```python
from build123d import *

# Parameters (mm, degrees)
F0_W           = 50.8
F0_H           = 43.18
F1_DEPTH       = 50.8
F3_D           = 6.35
F3_CBORE_D     = 9.525
F3_CBORE_DEPTH = 6.35
F5_D           = 7.9375
F6_SIZE        = 3.175


with BuildPart() as f1:
    # F0 (on Front) → F1 (new body)
    with BuildSketch(Plane.XZ):
        with Locations((25.4, -21.59)):
            Rectangle(F0_W, F0_H)
    extrude(amount=-F1_DEPTH)

    # F3 (through all)
    with Locations(Plane.XY):
        with Locations((7.1374, 7.1628), (7.1374, 43.6626), (43.6372, 43.6626), (43.6372, 7.1628)):
            CounterBoreHole(F3_D / 2, F3_CBORE_D / 2, F3_CBORE_DEPTH)

    # F5 (through all)
    with Locations(Plane.XY):
        with Locations((26.850944, 26.850944), (26.850944, 45.138944)):
            Hole(F5_D / 2)

    # F6
    f6_edges = [f1.edges().sort_by_distance(p)[0] for p in [
        (50.8, 50.8, -21.59),
        (50.8, 0, -21.59),
        (0, 50.8, -21.59),
        (0, 0, -21.59),
    ]]
    chamfer(f6_edges, length=F6_SIZE)


solid = f1.part
```
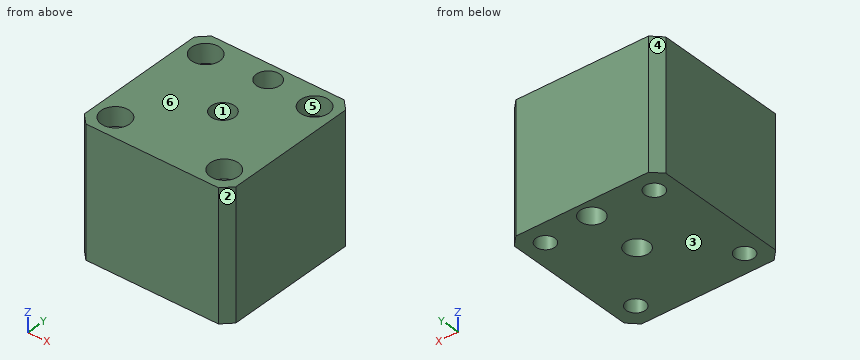
Read the model definition and answer for the solid it produces. Units are mm, in the model's axes. Face numbers are marked on the shaded views. A direction names the side the tool comes from. Coordinates: 2 decimals unless noted, no trailing zeros. Write each loop counter-clockwise with the first axis right and the second up, starting at its lowest first coordinate (ties: lowest second). Pieces come first, ordered by that corner, then holes. Notation, with made-up numbers: (-23.5, 81) - (-18.5, 81) arc R21 cw to (-18.5, 88) - close; hole circle Ø6 at (57.25, 31). An arc over 180 degrees is marked (long way). Answer as a JSON object with one key per item and string values. Group by question number.
1. A cutting plane is placed at B-B (z = -21). Give the number of separate pieces and of enclosed holes in the cut face, plus the area to 3 significant figures.
2. Which of the six approach directions +Z, -Z, +X, -X, +Y, -Y give full straight-line access (tool end or side, diameter ignored) to the marked faces 5 and 6?
3. A cutting plane is placed at A-A (x = 29.5). Determine the outline of the cut face in (y, z), plus the area to 3 significant figures.
4. Consider L1, parallel to X at y = 7, z = -36; L2, parallel to Y at x = 44.5, z = -13; L3, parallel to Y at x = 28.5, z = -27. Determine where each line is inside the solid, lowest interval first. Write a range as [from, to].
5. A cutting plane is placed at D-D (x = 9.5). Determine the outline of the cut face in (y, z), plus the area to 3 significant figures.
6. Each of these flat-tipped pins is pushed along its axis until it touches: P1, Ø9, axis at x = 26.85, y = 45.14, coming from the +Z side; P2, Ø3, axis at x = 6, y = 9, coming from the +Z side. Where does it stop, or does it pass through?
7. The mould has two halves that part along Y. Classify the marked faces 1, 2, 3 and 4: +Y half, -Y half, draft (parallel to the pull), parting line (faces both ways), or undercut.
8. A cutting plane is placed at C-C (x = 41.5). Determine the outline of the cut face in (y, z).
Worked out:
{
 "1": {"separate pieces": "1", "enclosed holes": "6", "area": "2,330 mm²"},
 "2": {"face 5": "+Z", "face 6": "+Z, +X, -X, +Y, -Y"},
 "3": {"outline": "(0, -43.18) - (23.9, -43.18) - (23.9, 0) - (0, 0) - close; (29.81, -43.18) - (42.18, -43.18) - (42.18, 0) - (29.81, 0) - close; (48.09, -43.18) - (50.8, -43.18) - (50.8, 0) - (48.09, 0) - close", "area": "1,680 mm²"},
 "4": {"L1": "x = [0, 3.97], [10.31, 40.47], [46.81, 50.8]", "L2": "y = [0, 4.11], [10.22, 40.61], [46.72, 50.8]", "L3": "y = [0, 23.24], [30.46, 41.53], [48.75, 50.8]"},
 "5": {"outline": "(0, -43.18) - (5.04, -43.18) - (5.04, -6.35) - (3.03, -6.35) - (3.03, 0) - (0, 0) - close; (9.28, -43.18) - (41.54, -43.18) - (41.54, -6.35) - (39.53, -6.35) - (39.53, 0) - (11.3, 0) - (11.3, -6.35) - (9.28, -6.35) - close; (45.78, -43.18) - (50.8, -43.18) - (50.8, 0) - (47.8, 0) - (47.8, -6.35) - (45.78, -6.35) - close", "area": "1,780 mm²"},
 "6": {"P1": "stops at z = 0", "P2": "stops at z = -6.35"},
 "7": {"face 1": "undercut", "face 2": "-Y half", "face 3": "draft", "face 4": "+Y half"},
 "8": {"outline": "(0, -43.18) - (4.81, -43.18) - (4.81, -6.35) - (2.91, -6.35) - (2.91, 0) - (0, 0) - close; (9.51, -43.18) - (41.31, -43.18) - (41.31, -6.35) - (39.41, -6.35) - (39.41, 0) - (11.42, 0) - (11.42, -6.35) - (9.51, -6.35) - close; (46.01, -43.18) - (50.8, -43.18) - (50.8, 0) - (47.92, 0) - (47.92, -6.35) - (46.01, -6.35) - close"}
}
